Build history of the part. All positions in model axes, mm. Give positions to 0.01 mm unless a question says otherwise; leave off trailing zeros. Loops run counter-clockwise (first coordinate to the right, second up) from the corner with the lowest first, then second, coordinate; pieces in that order, holes last. Notation, with made-up numbers: M -35,79 L -12,79 A9 ccw -12,92 Z; hole C -6,41 d6. An arc over 180 degrees is marked long. Put each result on its own line as item: value.
Autodesk Inventor part; units mm, degrees
ref_plane "YZ Plane" through (0, 0, 0) normal (1, 0, 0) x (0, 1, 0)
ref_plane "XZ Plane" through (0, 0, 0) normal (0, 1, 0) x (-1, 0, 0)
ref_plane "XY Plane" through (0, 0, 0) normal (0, 0, 1) x (1, 0, 0)
sketch "Sketch1" plane through (0, 0, 0) normal (0, 1, 0) x (-1, 0, 0)
  line L0 (-50, -10) -> (50, -10)
  line L1 (50, -10) -> (50, 10)
  line L2 (50, 10) -> (-50, 10)
  line L3 (-50, 10) -> (-50, -10)
  line L4 (-50, -10) -> (50, 10) construction
  line L5 (50, -10) -> (-50, 10) construction
  point P0 (0, 0)
  dimension "d0" = 100
  dimension "d1" = 20
extrude "Extrusion1" add sketch "Sketch1" along normal blind 5
sketch "Sketch2" plane through (0, 5, 0) normal (0, 1, 0) x (1, 0, 0)
  line L0 (-50, 10) -> (-50, -10)
  line L1 (-50, 0) -> (-40, 0)
  line L2 (50, -10) -> (50, 10)
  line L3 (50, 0) -> (40, 0)
  point P0 (0, 0)
  dimension "d4" = 10
  dimension "d5" = 10
hole "Hole1" at (-40, 5, 0) direction (0, -1, 0) diameter 4 depth 6
hole "Hole2" at (40, 5, 0) direction (0, -1, 0) diameter 4 depth 6
chamfer "Chamfer1" distance 2 angle 45 2 edges at (0, 0, 10) (0, 0, -10)
thread "Thread1"
thread "Thread2"
properties part number "Rail stand"
Q1. Mould opens along X. For faces 1 (the cylindrical face through (42, 2, 0)), 2 (the flat face through (50, 2, 0)), 3 (the flat face through (1, 3, -10)) say: pulls with the +X half, pulls with the -X half, needs draft (parallel to the pull), parting line crosses it, or undercut.
Here are the results:
face 1: undercut
face 2: pulls with the +X half
face 3: needs draft
Q2. Slice it at A-A (x = -40). List the corners of the cut face in (y, z), and give its area (3 significant figures).
Here are the results:
outline: M 0,-8 L 2,-10 L 5,-10 L 5,-2 L 0,-2 Z; M 0,2 L 5,2 L 5,10 L 2,10 L 0,8 Z
area: 76.0 mm²
Q3. Slice it at C-C (x = 6.5). List the corners of the cut face in (y, z), and give its area (3 significant figures).
Here are the results:
outline: M 0,-8 L 2,-10 L 5,-10 L 5,10 L 2,10 L 0,8 Z
area: 96.0 mm²
Q4. Slice it at B-B (z = 0). List the corners of the cut face in (x, y), and give its area (3 significant figures).
Here are the results:
outline: M -50,0 L -42,0 L -42,5 L -50,5 Z; M -38,0 L 38,0 L 38,5 L -38,5 Z; M 42,0 L 50,0 L 50,5 L 42,5 Z
area: 460 mm²
Q5. Probe line 1 (X direction, y = 3.9, z = 0); line 2 (Z direction, x = 40, y = 2.6); line 3 (Z direction, x = -40, y = 1.9). List the from-to ranges inside material, lowest first. Write a range as from..to.
Here are the results:
line 1: -50..-42, -38..38, 42..50
line 2: -10..-2, 2..10
line 3: -9.9..-2, 2..9.9
